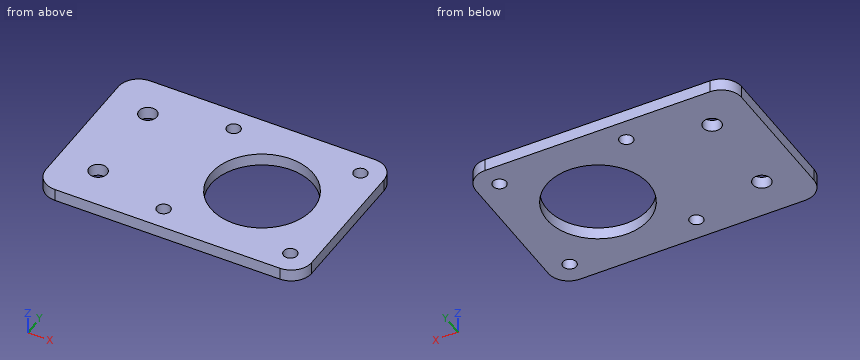
```python
from build123d import *

# Parameters (mm, degrees)
F0_W     = 65
F0_H     = 42
F1_DEPTH = 3
F3_D     = 3.3
F4_D     = 4.4
F5_D     = 25
F6_R     = 5


with BuildPart() as f1:
    # F0 (on Top) → F1 (new body)
    with BuildSketch(Plane.XY):
        with Locations((32.5, -21)):
            Rectangle(F0_W, F0_H)
    extrude(amount=F1_DEPTH)

    # F3 (through all)
    with Locations(Plane.XY.offset(3)):
        with Locations((28.5, -5.5), (28.5, -36.5), (59.5, -36.5), (59.5, -5.5)):
            Hole(F3_D / 2)

    # F4 (through all)
    with Locations(Plane.XY.offset(3)):
        with Locations((10, -10), (10, -32)):
            Hole(F4_D / 2)

    # F5 (through all)
    with Locations(Plane.XY.offset(3)):
        with Locations((44, -21)):
            Hole(F5_D / 2)

    # F6
    f6_edges = [f1.edges().sort_by_distance(p)[0] for p in [
        (0, -42, 1.5),
        (65, -42, 1.5),
        (65, 0, 1.5),
        (0, 0, 1.5),
    ]]
    fillet(f6_edges, radius=F6_R)


solid = f1.part
```
Check sheet for the modelled part. Datum: model origin and axes. Units: mm. Give positions to 0.01 mm unless a question says otherwise; leave off trailing zeros. Write each loop counter-clockwise with the first axis right and the second up, starting at its lowest first coordinate (ties: lowest second). Pieces come first, ordered by that corner, then holes. Notation, with made-up numbers: (30.5, -26.5) - (38.5, -26.5) arc R21 cw to (38.5, 3.5) - close; hole circle Ø2 at (-14.75, 56). An arc over 180 degrees is marked (long way). Answer as a JSON object with one key per item and string values. Group by question number.
1) Sectioned sample at C-C (x = 44.5). Record the cut outline in (y, z).
2) Sectioned sample at A-A (y = -21). Record the cut outline in (x, z), then the cut area to 3 significant figures.
3) Thickness scan on probe 1 along Y at (x, z) = (10, 2.1); probe 2 along Y at (x, z) = (59.5, 0.8); probe 3 along X at (y, z) = (-6.5, 0.35). Record the ranges inside material, lowest first. Write a range as from..to.
4) Depth check by flat-ended pin: P1, Ø4.5, axis at x = 28.5, y = -36.5, coming from the +Z side; P2, Ø2, axis at x = 59.5, y = -5.5, coming from the +Z side. Enter the tip coordinate at first touch or a pass-through.
5) Sectioned sample at D-D (x = 28.5). Record the cut outline in (y, z).
6) Sectioned sample at B-B (z = 1.4). Record the cut outline in (x, y), then the cut area to 3 significant figures.
Geometry results:
{
 "1": {"outline": "(-42, 0) - (-33.49, 0) - (-33.49, 3) - (-42, 3) - close; (-8.51, 0) - (0, 0) - (0, 3) - (-8.51, 3) - close"},
 "2": {"outline": "(0, 0) - (31.5, 0) - (31.5, 3) - (0, 3) - close; (56.5, 0) - (65, 0) - (65, 3) - (56.5, 3) - close", "area": "120 mm^2"},
 "3": {"probe 1": "y = -42..-34.2, -29.8..-12.2, -7.8..0", "probe 2": "y = -42..-38.15, -34.85..-7.15, -3.85..0", "probe 3": "x = 0..27.19, 29.81..58.19, 60.81..65"},
 "4": {"P1": "stops at z = 3", "P2": "passes through"},
 "5": {"outline": "(-42, 0) - (-38.15, 0) - (-38.15, 3) - (-42, 3) - close; (-34.85, 0) - (-7.15, 0) - (-7.15, 3) - (-34.85, 3) - close; (-3.85, 0) - (0, 0) - (0, 3) - (-3.85, 3) - close"},
 "6": {"outline": "(0, -37) arc R5 ccw to (5, -42) - (60, -42) arc R5 ccw to (65, -37) - (65, -5) arc R5 ccw to (60, 0) - (5, 0) arc R5 ccw to (0, -5) - close; hole circle Ø4.4 at (10, -32); hole circle Ø4.4 at (10, -10); hole circle Ø3.3 at (28.5, -36.5); hole circle Ø3.3 at (28.5, -5.5); hole circle Ø25 at (44, -21); hole circle Ø3.3 at (59.5, -36.5); hole circle Ø3.3 at (59.5, -5.5)", "area": "2,150 mm^2"}
}
